Design review of the part built by this model. Coordinates are the model's own, in mm. Face numbers are marked on the shaded views. A direction names the side the tool comes from. Coordinates: 2 decimals unless noted, no trailing zeros. Loops run counter-clockwise (first coordinate to the right, second up) from the corner with the lowest first, then second, coordinate; pieces in that order, holes last. Notation, with made-up numbers: (-18.75, 53.5) -> (-10.75, 53.5) arc R17 ccw to (-10.75, 61.5) -> close; hole circle Ø1 at (-13, 16). An arc over 180 degrees is marked (long way). Use a Markdown table: item, result. Add a question column.
Q1. For probe 1 along Y at (x, z) = (0, -6.5); probe 2 along X at (y, z) = (2.75, -5.5); probe 3 along Y at (x, z) = (1, -5.25), list the stretches that pass through material, from the lowest coordinate up.
Q2. Take a section at C-C on y = 0. Write out the cut boundary in (x, z) (1 decimal), plus the area to 3 significant figures.
Q3. Draft analysis for pull direction Y (two halves, no side actions). For the marked faces 1, 2, 3 and 4, state which applies: pulls with the +Y half, pulls with the -Y half, needs draft (parallel to the pull), parting line crosses it, or undercut.
Q4. For the marked faces 5, 6 and 7, list the 3-axis set-ups (+Z, -Z, +X, -X, +Y, -Y) from which the entire face can be reached by the end or side of a thin tool; tool diameter is ignored.
Q5. Clearance check with flat-ended pins moving along their axes: pin 1 Ø5 at (y, z) = (6.5, -7) entering from -X; pin 2 Ø1 at (y, z) = (-0.5, -7) entering from -X; pin 3 Ø3 at (x, z) = (5, -3) entering from +Y; pin 4 Ø4 at (x, z) = (9, -10.5) entering from +Y. State where each tip first meets the part, or that it passes through.
Q6. Take a section at A-A on z = -6.35. Write out the cut boundary in (x, y) (1 decimal), plus the area to 3 significant figures.
Q7. Take a section at B-B on x = 0. Count the separate pieces of the cut face and the enclosed holes in it, plus the area to 3 significant figures.
Q8. Take a section at D-D on z = -9.5. Write out the cut boundary in (x, y) (1 decimal).
from build123d import *

# Parameters (mm, degrees)
CHAMFER1_SIZE                  = 0.762
F_4_40_TAPPED_HOLE1_AT_2_COUNT = 2
F_4_40_TAPPED_HOLE1_AT_2_PITCH = 19.05
SKETCH4_W                      = 34.925
SKETCH4_H                      = 42.395859198
CUT_EXTRUDE1_DEPTH             = 0.8128


with BuildPart() as part:
    # Sketch1 → Revolve1 (revolve)
    with BuildSketch(Plane(origin=(0, 0, 0), x_dir=(0, 0, -1), z_dir=(1, 0, 0)), mode=Mode.PRIVATE) as revolve1_sk:
        Polygon((0, 3.9751), (11.684, 3.9751), (11.684, 5.55625), (12.7, 5.55625), (12.7, 14.1605), (0, 14.1605), align=None)
    revolve(revolve1_sk.sketch.rotate(Axis((0, 0, -16.392907801), (0, 0, -1)), 90), axis=Axis((0, 0, -16.392907801), (0, 0, -1)))

    # Chamfer1
    chamfer1_edges = [part.edges().sort_by_distance(p)[0] for p in [
        (-14.1605, 0, 0),
        (-14.1605, 0, -12.7),
    ]]
    chamfer(chamfer1_edges, length=CHAMFER1_SIZE)

    # Sketch2 → Cut-Revolve1 (revolve, cut)
    with BuildSketch(Plane.XY.offset(-6.35), mode=Mode.PRIVATE) as cut_revolve1_sk:
        Polygon((10.07745, 0), (10.07745, 7.9248), (11.8999, 7.9248), (11.8999, 20.6248), (7.9248, 20.6248), (7.9248, -19.869024768), (9.652, -18.871825383), (9.652, -0.245633672), align=None)
    revolve(cut_revolve1_sk.sketch.rotate(Axis((7.9248, -19.869024768, -6.35), (0, -1, 0)), 180), axis=Axis((7.9248, -19.869024768, -6.35), (0, -1, 0)), mode=Mode.SUBTRACT)

    # Sketch5 → 4-40 Tapped Hole1 (revolve, cut)
    with BuildSketch(Plane(origin=(0, 9.525, -12.7), x_dir=(0, 1, 0), z_dir=(1, 0, 0))):
        Polygon((0, 0), (0, 12.7), (1.651, 12.7), (1.1303, 12.1793), (1.1303, 0.5207), (1.651, 0), align=None)
    f_4_40_tapped_hole1 = revolve(axis=Axis((0, 9.525, -19.05), (0, 0, 1)), mode=Mode.SUBTRACT)

    # 4-40 Tapped Hole1 at 2: 4-40 Tapped Hole1 ×2
    with Locations(*[(0, -i * F_4_40_TAPPED_HOLE1_AT_2_PITCH, 0) for i in range(1, F_4_40_TAPPED_HOLE1_AT_2_COUNT)]):
        add(f_4_40_tapped_hole1, mode=Mode.SUBTRACT)

    # Sketch4 → Cut-Extrude1 (cut, symmetric)
    with BuildSketch(Plane(origin=(0, 0, 0), x_dir=(1, 0, 0), z_dir=(0, 1, 0))):
        with Locations((7.9375, 14.389486552)):
            Rectangle(SKETCH4_W, SKETCH4_H)
    extrude(amount=CUT_EXTRUDE1_DEPTH, both=True, mode=Mode.SUBTRACT)


solid = part.part
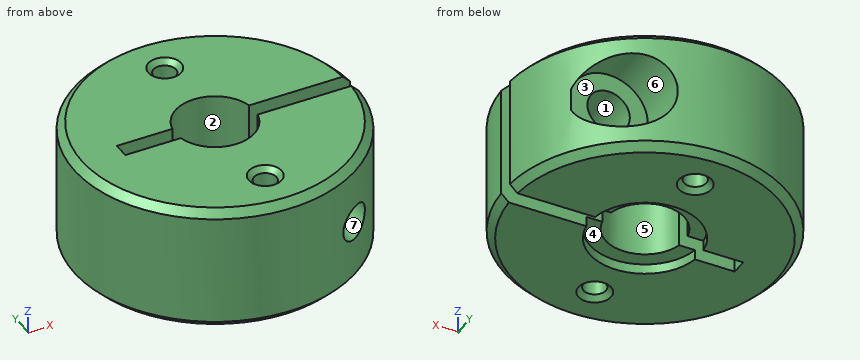
Answer list:
| question | item | result |
|---|---|---|
| 1 | probe 1 | -14.16 to -10.66, -8.39 to -3.98, 3.98 to 8.39, 10.66 to 14.16 |
| 1 | probe 2 | -13.89 to -2.87, 2.87 to 5.95, 9.9 to 13.89 |
| 1 | probe 3 | -14.13 to -10.05, -9 to -3.85, 3.85 to 9, 10.05 to 14.13 |
| 2 | outline | (-14.2, -11.9) -> (-13.4, -12.7) -> (-9.5, -12.7) -> (-9.5, 0) -> (-13.4, 0) -> (-14.2, -0.8) -> close |
| 2 | area | 58.3 mm² |
| 3 | face 1 | needs draft |
| 3 | face 2 | undercut |
| 3 | face 3 | pulls with the +Y half |
| 3 | face 4 | undercut |
| 4 | face 5 | +Z, -Z |
| 4 | face 6 | +Y |
| 4 | face 7 | +Y, -Y |
| 5 | pin 1 | x = -13.58 |
| 5 | pin 2 | x = -14.16 |
| 5 | pin 3 | y = 13.72 |
| 5 | pin 4 | y = 12.31 |
| 6 | outline | (-9.5, -0.8) -> (-9.5, 0.8) -> (-3.9, 0.8) arc R4 cw to (3.9, 0.8) -> (5.8, 0.8) -> (5.8, 7.9) -> (3.9, 7.9) -> (3.9, 13.6) arc R14.2 ccw (long way) to (6.2, -12.7) -> (6.2, -0.8) -> (3.9, -0.8) arc R4 cw to (-3.9, -0.8) -> close; (9.7, -10.4) arc R14.2 ccw to (14.1, -0.8) -> (9.7, -0.8) -> close; (10.1, 0.8) -> (14.1, 0.8) arc R14.2 ccw to (11.7, 7.9) -> (10.1, 7.9) -> close; hole circle Ø2.3 at (0, -9.5); hole circle Ø2.3 at (0, 9.5) |
| 6 | area | 451 mm² |
| 7 | separate pieces | 4 |
| 7 | enclosed holes | 0 |
| 7 | area | 196 mm² |
| 8 | outline | (-9.5, -0.8) -> (-9.5, 0.8) -> (-3.9, 0.8) arc R4 cw to (3.9, 0.8) -> (14.1, 0.8) arc R14.2 ccw to (10.3, 9.7) -> (10.3, 7.9) -> (5.5, 7.9) -> (5.5, 13) arc R14.2 ccw (long way) to (14.1, -0.8) -> (3.9, -0.8) arc R4 cw to (-3.9, -0.8) -> close; hole circle Ø2.3 at (0, -9.5); hole circle Ø2.3 at (0, 9.5) |
